Source: CAD feature listing. Evaluate the final solid. Frame: model axes, mm. A direction names the side the tool comes from. Coordinates: 2 decimals unless noted, no trailing zeros. Order: outer loops, then holes, each group sorted by start corner. A loop starts at its lowest first (then second) coordinate and runs counter-clockwise, first axis right, second up.
Item 1: Mould query, pull axis X, two halves, no side actions, for faces 1 (the flat face through (-40.5, 20, 6)), 2 (the cylindrical face through (20.68, 5.59, 9.34)), 3 (the flat face through (-26, -10, 6)). Classes: released by +X, released by -X, zero draft, split by the parting line, or undercut.
Item 2: Section B-B on x = -3.5. Return the cut outline in (y, z).
Item 3: Reachability of faces 4 (the flat face through (18, 2, 6.6)), 5 (the cylindrical face through (-36.8, 29.02, 6.73)), 6 (the cylindrical face through (36.8, -4.25, 5.75)) from +Z, -Z, +X, -X, +Y, -Y: full face, straight path, thin tool, end or side. Return the list, or none.
Item 4: Section C-C on z = 10. Return the cut outline in (x, y), then the cut area to 3 significant figures.
Item 5: Ray query, line 1 (Y direction, x = -15.5, z = 10.75); line 2 (Y direction, x = 38, z = 7); line 3 (Z direction, x = -35, y = 43.5). Return the intervals inside material, ascending.
Item 6: Contact query for flat-ended pins moving along their axis: P1, Ø24, axis at x = 3.5, y = -39.5, coming from the -Z side; P2, Ø3.5, axis at x = 15.91, y = 4.09, coming from the +Z side; P3, Ø1.5, axis at y = -34.2, z = 7, coming from the -X side; P4, Ø2, axis at y = -4.2, z = 7, coming from the -X side. Output: stop coordinate, or through.
Item 7: Section D-D on y = -15.5. Return the cut outline in (x, z), then the cut area to 3 significant figures.
Item 8: Section A-A on y = 20. Return the cut outline in (x, z).
from build123d import *

# Parameters (mm, degrees)
SKETCH_1_W                   = 81
SKETCH_1_H                   = 100
EXTRUDE_1_DEPTH              = 12
SKETCH_2_R                   = 13
CUT_EXTRUDE_1_DEPTH          = 66.454182448
HOLE_WIZARD_M5_1_D           = 5.5
HOLE_WIZARD_M5_1_CBORE_D     = 10
HOLE_WIZARD_M5_1_CBORE_DEPTH = 5.4
HOLE_WIZARD_M3_1_AT_2_COUNT  = 2
HOLE_WIZARD_M3_1_AT_2_PITCH  = 15.7
HOLE_WIZARD_M3_1_AT_3_COUNT  = 2
HOLE_WIZARD_M3_1_AT_3_PITCH  = 47.7
HOLE_WIZARD_M3_1_AT_4_COUNT  = 2
HOLE_WIZARD_M3_1_AT_4_PITCH  = 77.7
SKETCH_9_R                   = 16.5
CUT_EXTRUDE_2_DEPTH          = 2
SKETCH_10_W                  = 81
SKETCH_10_H                  = 30
CUT_EXTRUDE_3_DEPTH          = 2
SKETCH_11_W                  = 60
SKETCH_11_H                  = 20
CUT_EXTRUDE_4_DEPTH          = 84
FILLET_1_R                   = 2
HOLE_WIZARD_M3_2_D           = 2.5
HOLE_WIZARD_M3_2_DEPTH       = 7.5
HOLE_WIZARD_M3_2_TIP         = 0.751075774


with BuildPart() as part:
    # 草图1 → 凸台-拉伸1 (new body)
    with BuildSketch(Plane.XY):
        Rectangle(SKETCH_1_W, SKETCH_1_H)
    extrude(amount=EXTRUDE_1_DEPTH)

    # 草图2 → 切除-拉伸1 (cut, through all)
    with BuildSketch(Plane(origin=(0, 0, 0), x_dir=(-1, 0, 0), z_dir=(0, 0, -1))):
        with Locations((0, 20)):
            Circle(SKETCH_2_R)
    extrude(amount=-CUT_EXTRUDE_1_DEPTH, mode=Mode.SUBTRACT)

    # M5 六角凹头螺钉的柱形沉头孔1 (through all)
    with Locations(Plane.XY.offset(12)):
        with Locations((-15.909902577, 35.909902577), (15.909902577, 35.909902577), (15.909902577, 4.090097423), (-15.909902577, 4.090097423), (0, 20)):
            CounterBoreHole(HOLE_WIZARD_M5_1_D / 2, HOLE_WIZARD_M5_1_CBORE_D / 2, HOLE_WIZARD_M5_1_CBORE_DEPTH)

    # 草图7 → M3 螺纹孔1 (revolve, cut)
    with BuildSketch(Plane(origin=(-40.5, 43.5, 7), x_dir=(0, 0, 1), z_dir=(0, 1, 0))):
        Polygon((0, 0), (0, 8.251075774), (1.25, 7.5), (1.25, 0), align=None)
    hole_wizard_m3_1 = revolve(axis=Axis((-46.85, 43.5, 7), (1, 0, 0)), mode=Mode.SUBTRACT)

    # M3 螺纹孔1 at 2: M3 螺纹孔1 ×2
    with Locations(*[(0, -i * HOLE_WIZARD_M3_1_AT_2_PITCH, 0) for i in range(1, HOLE_WIZARD_M3_1_AT_2_COUNT)]):
        add(hole_wizard_m3_1, mode=Mode.SUBTRACT)

    # M3 螺纹孔1 at 3: M3 螺纹孔1 ×2
    with Locations(*[(0, -i * HOLE_WIZARD_M3_1_AT_3_PITCH, 0) for i in range(1, HOLE_WIZARD_M3_1_AT_3_COUNT)]):
        add(hole_wizard_m3_1, mode=Mode.SUBTRACT)

    # M3 螺纹孔1 at 4: M3 螺纹孔1 ×2
    with Locations(*[(0, -i * HOLE_WIZARD_M3_1_AT_4_PITCH, 0) for i in range(1, HOLE_WIZARD_M3_1_AT_4_COUNT)]):
        add(hole_wizard_m3_1, mode=Mode.SUBTRACT)

    # 镜向1: M3 螺纹孔1 across plane
    add(hole_wizard_m3_1.mirror(Plane(origin=(0, 0, 0), x_dir=(0, 0, 1), z_dir=(1, 0, 0))), mode=Mode.SUBTRACT)

    # 镜向1 copy 1 sketch → 镜向1 copy 1 (revolve, cut)
    with BuildSketch(Plane(origin=(40.5, 27.8, 7), x_dir=(0, 0, 1), z_dir=(0, 1, 0))):
        Polygon((0, 0), (0, -8.251075774), (1.25, -7.5), (1.25, 0), align=None)
    revolve(axis=Axis((46.85, 27.8, 7), (1, 0, 0)), mode=Mode.SUBTRACT)

    # 镜向1 copy 2 sketch → 镜向1 copy 2 (revolve, cut)
    with BuildSketch(Plane(origin=(40.5, -4.2, 7), x_dir=(0, 0, 1), z_dir=(0, 1, 0))):
        Polygon((0, 0), (0, -8.251075774), (1.25, -7.5), (1.25, 0), align=None)
    revolve(axis=Axis((46.85, -4.2, 7), (1, 0, 0)), mode=Mode.SUBTRACT)

    # 镜向1 copy 3 sketch → 镜向1 copy 3 (revolve, cut)
    with BuildSketch(Plane(origin=(40.5, -34.2, 7), x_dir=(0, 0, 1), z_dir=(0, 1, 0))):
        Polygon((0, 0), (0, -8.251075774), (1.25, -7.5), (1.25, 0), align=None)
    revolve(axis=Axis((46.85, -34.2, 7), (1, 0, 0)), mode=Mode.SUBTRACT)

    # 草图9 → 切除-拉伸2 (cut)
    with BuildSketch(Plane(origin=(0, 0, 0), x_dir=(-1, 0, 0), z_dir=(0, 0, -1))):
        with Locations((0, 20)):
            Circle(SKETCH_9_R)
    extrude(amount=-CUT_EXTRUDE_2_DEPTH, mode=Mode.SUBTRACT)

    # 草图10 → 切除-拉伸3 (cut)
    with BuildSketch(Plane(origin=(0, 0, 0), x_dir=(-1, 0, 0), z_dir=(0, 0, -1))):
        with Locations((0, -35)):
            Rectangle(SKETCH_10_W, SKETCH_10_H)
    extrude(amount=-CUT_EXTRUDE_3_DEPTH, mode=Mode.SUBTRACT)

    # 草图11 → 切除-拉伸4 (cut)
    with BuildSketch(Plane(origin=(0, 0, 0), x_dir=(-1, 0, 0), z_dir=(0, 0, -1))):
        with Locations((40.5, -20)):
            Rectangle(SKETCH_11_W, SKETCH_11_H)
    extrude(amount=-CUT_EXTRUDE_4_DEPTH, mode=Mode.SUBTRACT)

    # 圆角1
    fillet_1_edges = [part.edges().sort_by_distance(p)[0] for p in [
        (-10.5, -10, 6),
        (-10.5, -30, 7),
    ]]
    fillet(fillet_1_edges, radius=FILLET_1_R)

    # M3 螺纹孔2
    with Locations(Plane.XY.offset(12)):
        with Locations((7.5, -27.5), (-7.5, -27.5)):
            Hole(HOLE_WIZARD_M3_2_D / 2, depth=HOLE_WIZARD_M3_2_DEPTH)
            with Locations((0, 0, -(HOLE_WIZARD_M3_2_DEPTH + HOLE_WIZARD_M3_2_TIP / 2))):  # 118° drill point
                Cone(0, HOLE_WIZARD_M3_2_D / 2, HOLE_WIZARD_M3_2_TIP, mode=Mode.SUBTRACT)


solid = part.part
Answer list:
1. face 1: released by -X
1. face 2: undercut
1. face 3: zero draft
2. outline: (-50, 2) - (-20, 2) - (-20, 0) - (3.88, 0) - (3.88, 2) - (7.48, 2) - (7.48, 12) - (-50, 12) - close; (32.52, 2) - (36.12, 2) - (36.12, 0) - (50, 0) - (50, 12) - (32.52, 12) - close
3. face 4: +Z
3. face 5: -X
3. face 6: +X
4. outline: (-40.5, -50) - (40.5, -50) - (40.5, 50) - (-40.5, 50) - (-40.5, -10) - (-12.5, -10) arc R2 cw to (-10.5, -12) - (-10.5, -28) arc R2 cw to (-12.5, -30) - (-40.5, -30) - close; hole circle Ø10 at (-15.91, 4.09); hole circle Ø10 at (-15.91, 35.91); hole circle Ø26 at (0, 20); hole circle Ø2.5 at (-7.5, -27.5); hole circle Ø2.5 at (7.5, -27.5); hole circle Ø10 at (15.91, 4.09); hole circle Ø10 at (15.91, 35.91)
4. area: 6,650 mm2
5. line 1: y = -50 to -30, -10 to -0.89, 9.07 to 30.93, 40.89 to 50
5. line 2: y = -50 to -35.45, -32.95 to -5.45, -2.95 to 26.55, 29.05 to 42.25, 44.75 to 50
5. line 3: z = 0 to 5.75, 8.25 to 12
6. P1: stops at z = 2
6. P2: passes through
6. P3: stops at x = -32.7
6. P4: stops at x = -32.85
7. outline: (-10.5, 0) - (40.5, 0) - (40.5, 12) - (-10.5, 12) - close
7. area: 612 mm2
8. outline: (-40.5, 0) - (-16.5, 0) - (-16.5, 2) - (-13, 2) - (-13, 12) - (-40.5, 12) - close; (13, 2) - (16.5, 2) - (16.5, 0) - (40.5, 0) - (40.5, 12) - (13, 12) - close
